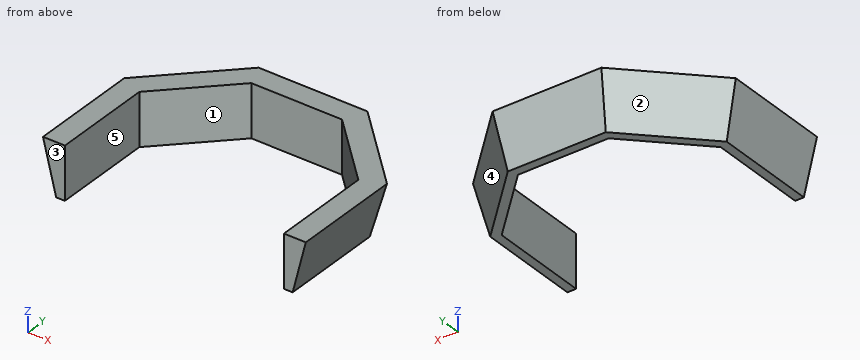
```python
from build123d import *

# Parameters (mm, degrees)
F1_DEPTH = 12
F2_SIZE2 = 11.99999
F2_SIZE  = 2.99999


# Not quite as in the source:
# - a fillet or chamfer is up to 0.001 mm smaller than in the source, because OpenCascade refuses the exact size


with BuildPart() as f1:
    # F0 (on Top) → F1 (new body)
    with BuildSketch(Plane.XY):
        Polygon((12.4264068712, 30), (-12.4264068712, 30), (-30, 12.4264068712), (-30, -12.4264068712), (-25, -12.4264068712), (-25, 10.3553390593), (-10.3553390593, 25), (10.3553390593, 25), (25, 10.3553390593), (25, -12.4264068712), (30, -12.4264068712), (30, 12.4264068712), align=None)
    extrude(amount=F1_DEPTH)

    # F2 (size 3 and 12 in the source; OpenCascade refuses exactly that, so slightly less here)
    f2_edges = [f1.edges().sort_by_distance(p)[0] for p in [
        (-30, 0, 0),
        (-21.213203, 21.213203, 0),
        (0, 30, 0),
        (21.213203, 21.213203, 0),
        (30, 0, 0),
    ]]
    f2_side = f1.faces().sort_by_distance((0, 29.265153, 0))[0]
    chamfer(f2_edges, length=F2_SIZE, length2=F2_SIZE2, reference=f2_side)


solid = f1.part
```
Geometry: final body of the model. Coordinates: model frame, mm. Face numbers are marked on the shaded views. A direction names the side the tool comes from. Round coordinates to 2 decimals unless told otherwise and drop trailing zeros. Write each loop counter-clockwise with the first axis right and the second up, starting at its lowest first coordinate (ties: lowest second). Pieces come first, ordered by that corner, then holes.
Item 1: Material intervals for L1, parallel to X at y = -4.5, z = 5.25; L2, parallel to X at y = 8.5, z = 4; L3, parallel to Y at x = -11.5, z = 3.5 (3 decimals), sorted ascending.
Item 2: Mould query, pull axis X, two halves, no side actions, for the marked faces 3, 4 and 5. Classes: +X half, -X half, draft (parallel to the pull), parting line (faces both ways), or undercut.
Item 3: Section query C-C (z = 11). Return loops of the section in (x, y), plus the area to 3 significant figures.
Item 4: Set-up query: the marked faces 1 and 2. Return all of +Z, -Z, +X, -X, +Y, -Y with unobstructed straight access to the full face (end or side cutting, diameter ignored); none if empty.
Item 5: Pin query (flat end, axial travel): P1, Ø6, axis at x = 2.5, z = 6, coming from the -Y side; P2, Ø6, axis at y = 3.5, z = 3.5, coming from the +X side (3 decimals); P3, Ø3.5, axis at y = 1.5, z = 6.5, coming from the -X side. Return the tip coordinate at first contact, or that it passes through.
Completed:
1. L1: x = -28.31 to -25, 25 to 28.31
1. L2: x = -28 to -25, 25 to 28
1. L3: y = 23.855 to 27.875
2. face 3: draft
2. face 4: +X half
2. face 5: undercut
3. outline: (-29.75, -12.43) - (-25, -12.43) - (-25, 10.36) - (-10.36, 25) - (10.36, 25) - (25, 10.36) - (25, -12.43) - (29.75, -12.43) - (29.75, 12.32) - (12.32, 29.75) - (-12.32, 29.75) - (-29.75, 12.32) - close
3. area: 549 mm2
4. face 1: +Z, -Z, -Y
4. face 2: -Z, -X, +Y
5. P1: stops at y = 25
5. P2: stops at x = 28.625
5. P3: stops at x = -29.06
